Work out the finished part from the listing and answer in its coordinate system (mm). Face numbers are marked on the shaded views. A direction names the side the tool comes from. Coordinates: 2 decimals unless noted, no trailing zeros. Loops run counter-clockwise (first coordinate to the right, second up) from the corner with the lowest first, then second, coordinate; pieces in that order, holes last.
```python
from build123d import *

# Parameters (mm, degrees)
F1_DEPTH = 19.1008
F3_DEPTH = 76.2
F4_T     = -2.54
F5_R     = 22.0345
F6_DEPTH = 6.35
F7_R     = 6.35
F8_T     = -4.699
F9_R     = 5.08


with BuildPart() as f1:
    # F0 (on Top) → F1 (new body)
    with BuildSketch(Plane.XY):
        with BuildLine():
            ThreePointArc((-50.7750985182, 50.8), (-76.1750985182, 25.4), (-50.7750985182, 0))
            Line((-50.7750985182, 0), (12.7249014818, 0))
            Line((12.7249014818, 0), (12.7249014818, 50.8))
            Line((12.7249014818, 50.8), (-50.7750985182, 50.8))
        make_face()
    extrude(amount=F1_DEPTH)

    # F2 (on face) → F3 (cut)
    with BuildSketch(Plane.XZ):
        Polygon((-76.1750985182, 16.51), (12.7249014818, 19.1008), (-76.1750985182, 19.1008), align=None)
    extrude(amount=-F3_DEPTH, mode=Mode.SUBTRACT)

    # F4
    f4_openings = [f1.faces().sort_by_distance(p)[0] for p in [
        (-29.192225, 25.4, 0),
    ]]
    offset(amount=F4_T, openings=f4_openings, kind=Kind.INTERSECTION)

    # F5 (on face) → F6 (join)
    with BuildSketch(Plane(origin=(-0.4713899101, 0, 16.1751439753), x_dir=(0.9995756172, 0, 0.0291304894), z_dir=(0.0291304894, 0, -0.9995756172))):
        with Locations((-18.9927711198, -25.4)):
            Circle(F5_R)
    extrude(amount=F6_DEPTH)

    # F7
    f7_edges = [f1.edges().sort_by_distance(p)[0] for p in [
        (12.724901, 50.8, 9.5504),
        (12.724901, 0, 9.5504),
    ]]
    fillet(f7_edges, radius=F7_R)

    # F8
    f8_openings = [f1.faces().sort_by_distance(p)[0] for p in [
        (-19.271122, 25.4, 9.27457),
    ]]
    offset(amount=F8_T, openings=f8_openings)

    # F9
    f9_edges = [f1.edges().sort_by_distance(p)[0] for p in [
        (10.184901, 2.54, 8.242849),
        (10.184901, 48.26, 8.242849),
    ]]
    fillet(f9_edges, radius=F9_R)


solid = f1.part
```
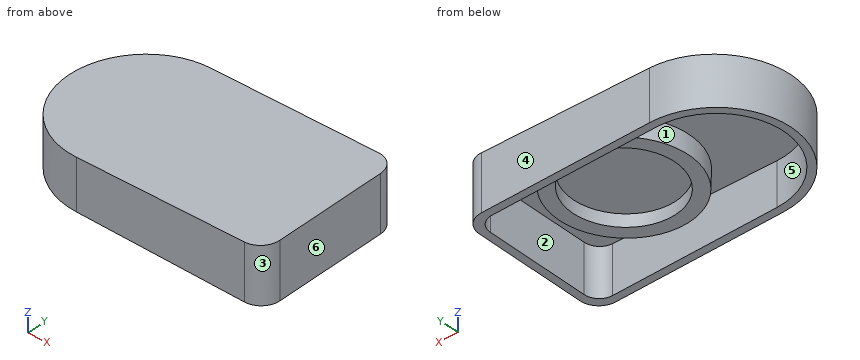
1. A cutting plane is placed at B-B, the plane x = -54. Give the vertices of the cut face in (y, z), then the cut area to 3 significant figures.
2. Each of these flat-tipped pins is pushed along its axis until it touches: P1, Ø8, axis at y = 24, z = 4.5, coming from the -X side; P2, Ø8, axis at x = -7.5, y = 38, coming from the +Z side; P3, Ø1, axis at x = -9, y = 8, coming from the +Z side; P4, Ø1, axis at x = -43.5, y = 41, coming from the -Z side. Where does it stop, or does it pass through?
3. A cutting plane is placed at C-C, the plane y = 40.5. Give the vertices of the cut face in (x, z) (3 decimals).
4. Straight lines are drawn through the part: probe 1 along Y at (x, z) = (-33, 9); probe 2 along Y at (x, z) = (-47.5, 4.5); probe 3 along Y at (x, z) = (-34, 10.25). For each, find the intervals that lie inside material, in ascending order.
5. Determine the mould class of the marked faces 1, 2, 3 and 4 for opening direction Y: released by +Y, released by -Y, zero draft, split by the parting line, or undercut.
6. A cutting plane is placed at A-A, the plane y = 15. Give the vertices of the cut face in (x, z), then the cut area to 3 significant figures.
7. For the marked faces 5 and 6, determine the directions among +Z, -Z, +X, -X, +Y, -Y from which every point of the face is accessible in a straight line to the end or side of a thin tool.
Answers below:
1. outline: (0.21, 0) - (2.77, 0) - (2.77, 14.62) - (48.03, 14.62) - (48.03, 0) - (50.59, 0) - (50.59, 17.16) - (0.21, 17.16) - close
1. area: 203 mm2
2. P1: stops at x = -76.18
2. P2: stops at z = 18.63
2. P3: stops at z = 18.48
2. P4: stops at z = 14.91
3. outline: (-71.199, 0) - (-67.938, 0) - (-67.938, 14.209) - (-35.496, 15.154) - (-35.311, 8.807) - (-27.783, 9.027) - (-27.905, 13.216) - (-10.882, 13.712) - (-10.759, 9.523) - (-3.231, 9.742) - (-3.416, 16.089) - (10.185, 16.486) - (10.185, 0) - (12.725, 0) - (12.725, 19.101) - (-71.199, 16.655) - close
4. probe 1: y = 0 to 2.54, 8.17 to 14.82, 35.98 to 42.63, 48.26 to 50.8
4. probe 2: y = 0 to 2.54, 48.26 to 50.8
4. probe 3: y = 0 to 2.54, 8.98 to 16.2, 34.6 to 41.82, 48.26 to 50.8
5. face 1: undercut
5. face 2: undercut
5. face 3: released by -Y
5. face 4: released by +Y
6. outline: (-73.95, 0) - (-71.13, 0) - (-71.13, 14.12) - (-38.87, 15.06) - (-38.69, 8.71) - (-33.13, 8.87) - (-33.26, 13.06) - (-5.53, 13.87) - (-5.41, 9.68) - (0.15, 9.84) - (-0.04, 16.19) - (10.18, 16.49) - (10.18, 0) - (12.72, 0) - (12.72, 19.1) - (-73.95, 16.57) - close
6. area: 432 mm2
7. face 5: -Z
7. face 6: +Z, -Z, +X, +Y, -Y
